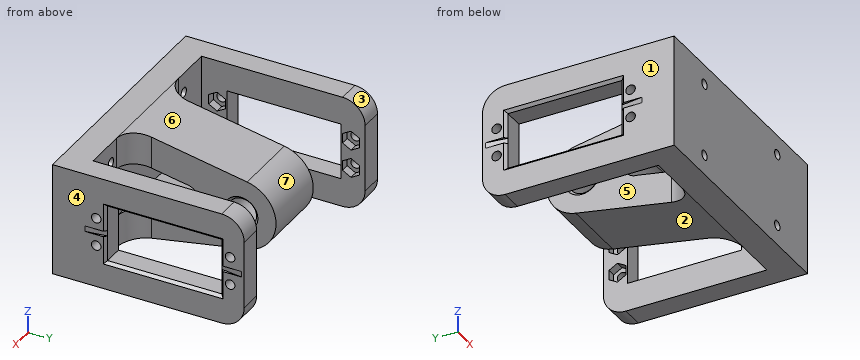
from build123d import *

# Parameters (mm, degrees)
SKETCH_1_W             = 8
SKETCH_1_H             = 58
SKETCH_1_W_2           = 12
EXTRUDE_1_DEPTH        = 20
SKETCH_3_R             = 1.7
SKETCH_3_W             = 20
SKETCH_3_H             = 40.5
CUT_EXTRUDE_1575_DEPTH = 8
SKETCH_2_R             = 5.05
CUT_EXTRUDE_2513_DEPTH = 12
CUT_EXTRUDE_2852_DEPTH = 1
SKETCH_5_R             = 1.7
CUT_EXTRUDE_3257_DEPTH = 3
SKETCH_6_R             = 1.7
CUT_EXTRUDE_5_DEPTH    = 10
FILLET_1_R             = 8
CHAMFER_1_SIZE         = 1


with BuildPart() as part:
    # Эскиз1 → Бобышка-Вытянуть1 (new body, symmetric)
    with BuildSketch(Plane.XY):
        Polygon((0, -10), (0, 0), (-12, 0), (-35, 0), (-43, 0), (-43, -10), align=None)
        with Locations((-39, 29)):
            Rectangle(SKETCH_1_W, SKETCH_1_H)
        with Locations((-6, 29)):
            Rectangle(SKETCH_1_W_2, SKETCH_1_H)
    extrude(amount=EXTRUDE_1_DEPTH, both=True)

    # Эскиз3 → Cut-Extrude 1575 (cut)
    with BuildSketch(Plane.ZY.offset(43)):
        with Locations((-5, 53)):
            Circle(SKETCH_3_R)
        with Locations((5, 53)):
            Circle(SKETCH_3_R)
        with Locations((-5, 5.5)):
            Circle(SKETCH_3_R)
        with Locations((5, 5.5)):
            Circle(SKETCH_3_R)
        with Locations((0, 29.25)):
            Rectangle(SKETCH_3_W, SKETCH_3_H)
    extrude(amount=-CUT_EXTRUDE_1575_DEPTH, mode=Mode.SUBTRACT)

    # Эскиз2 → Cut-Extrude 2513 (cut)
    with BuildSketch(Plane.ZY.offset(12)):
        with BuildLine():
            Line((-20, 58), (-20, 0))
            Line((-20, 0), (-12.294865589, 42.005278284))
            ThreePointArc((-12.294865589, 42.005278284), (0, 52.25), (12.294865589, 42.005278284))
            Line((12.294865589, 42.005278284), (20, 0))
            Line((20, 0), (20, 58))
            Line((20, 58), (-20, 58))
        make_face()
        with BuildLine():
            Line((-5, 20), (-8.668650572, 0))
            Line((-8.668650572, 0), (8.668650572, 0))
            Line((8.668650572, 0), (5, 20))
            ThreePointArc((5, 20), (0, 25), (-5, 20))
        make_face()
        with Locations((0, 39.75)):
            Circle(SKETCH_2_R)
    extrude(amount=-CUT_EXTRUDE_2513_DEPTH, mode=Mode.SUBTRACT)

    # Эскиз4 → Cut-Extrude 2852 (cut, symmetric)
    with BuildSketch(Plane.XY):
        Polygon((-42, 49.5), (-43, 49.5), (-43, 57), align=None)
        Polygon((-43, 9), (-43, 1.5), (-42, 9), align=None)
    extrude(amount=CUT_EXTRUDE_2852_DEPTH, both=True, mode=Mode.SUBTRACT)

    # Эскиз5 → Cut-Extrude 3257 (cut)
    with BuildSketch(Plane(origin=(-35, 0, 0), x_dir=(0, 0, -1), z_dir=(1, 0, 0))):
        Polygon((-6.732050808, 56), (-8.464101615, 53), (-6.732050808, 50), (-3.267949192, 50), (-1.535898385, 53), (-3.267949192, 56), align=None)
        with Locations((-5, 53)):
            Circle(SKETCH_5_R, mode=Mode.SUBTRACT)
        Polygon((1.535898385, 53), (3.267949192, 50), (6.732050808, 50), (8.464101615, 53), (6.732050808, 56), (3.267949192, 56), align=None)
        with Locations((5, 53)):
            Circle(SKETCH_5_R, mode=Mode.SUBTRACT)
        Polygon((-6.732050808, 8.5), (-8.464101615, 5.5), (-6.732050808, 2.5), (-3.267949192, 2.5), (-1.535898385, 5.5), (-3.267949192, 8.5), align=None)
        with Locations((-5, 5.5)):
            Circle(SKETCH_5_R, mode=Mode.SUBTRACT)
        Polygon((1.535898385, 5.5), (3.267949192, 2.5), (6.732050808, 2.5), (8.464101615, 5.5), (6.732050808, 8.5), (3.267949192, 8.5), align=None)
        with Locations((5, 5.5)):
            Circle(SKETCH_5_R, mode=Mode.SUBTRACT)
    extrude(amount=-CUT_EXTRUDE_3257_DEPTH, mode=Mode.SUBTRACT)

    # Эскиз6 → Вырез-Вытянуть5 (cut)
    with BuildSketch(Plane(origin=(0, 0, 0), x_dir=(1, 0, 0), z_dir=(0, 1, 0))):
        with Locations((-23.5, 13)):
            Circle(SKETCH_6_R)
        with Locations((-23.5, -13)):
            Circle(SKETCH_6_R)
    extrude(amount=-CUT_EXTRUDE_5_DEPTH, mode=Mode.SUBTRACT)

    # Скругление1
    fillet_1_edges = [part.edges().sort_by_distance(p)[0] for p in [
        (-39, 58, -20),
        (-12, 0, 14.334325286),
        (-39, 58, 20),
        (-12, 0, -14.334325286),
    ]]
    fillet(fillet_1_edges, radius=FILLET_1_R)

    # Фаска1
    chamfer_1_edges = [part.edges().sort_by_distance(p)[0] for p in [
        (-12, 39.75, -5.05),
        (-43, 9, 5.5),
        (-43, 49.5, 5.5),
        (-43, 29.25, 10),
        (-43, 9, -5.5),
        (-43, 49.5, -5.5),
        (-43, 29.25, -10),
    ]]
    chamfer(chamfer_1_edges, length=CHAMFER_1_SIZE)

    # Зеркальное отражение2: part across face


with BuildPart() as part_1:
    add(part.part)
    add(part.part.mirror(Plane(origin=(0, 17.029159437, 0), x_dir=(0, 0, 1), z_dir=(1, 0, 0))))


solid = part_1.part
The model under review builds one solid part; all positions refer to its coordinate system, in mm. Face numbers are marked on the shaded views. A direction names the side the tool comes from. Round coordinates to 2 decimals unless told otherwise and drop trailing zeros. Loops run counter-clockwise (first coordinate to the right, second up) from the corner with the lowest first, then second, coordinate; pieces in that order, holes last. Notation, with made-up numbers: (75, 62) -> (86, 62) arc R23 ccw to (86, 78) -> close; hole circle Ø3 at (70.25, 10.5). An arc over 180 degrees is marked (long way). Return JSON: item names as keys, results as strings.
(1) Add section D-D on z = 17. Write out the cut boundary in (x, y) (3 decimals), plus the area to 3 significant figures.
Solved:
{"outline": "(-43, -10) -> (43, -10) -> (43, 56.245) -> (35, 56.245) -> (35, 0) -> (20, 0) arc R8 cw to (12, 8) -> (12, 16.355) -> (-12, 16.355) -> (-12, 8) arc R8 cw to (-20, 0) -> (-35, 0) -> (-35, 56.245) -> (-43, 56.245) -> close", "area": "2,180 mm2"}
(2) For pin 1 (8 mm diameter, centred on y = 13.5, z = -4, fed in from -X); pin 2 (2.5 mm diameter, centred on x = -23.5, z = -13, fed in from +Y); pin 3 (1.5 mm diameter, centred on x = -22.5, z = -7.5, fed in from +Y), all flat-tipped, find the tip position at first contact; note any pin that passes through.
Solved:
{"pin 1": "x = -12", "pin 2": "through", "pin 3": "y = 0"}
(3) Add section A-A on z = 0. State how many separate pieces and enclosed holes the cut face has, plus the area to 3 significant figures.
Solved:
{"separate pieces": "5", "enclosed holes": "0", "area": "1,530 mm2"}
(4) For the marked faces 5, 6 and 7, list the 3-axis set-ups (+Z, -Z, +X, -X, +Y, -Y) from which the entire face can be reached by the end or side of a thin tool; tool diameter is ignored.
Solved:
{"face 5": "+Z, -Z, +Y", "face 6": "+Z, +Y", "face 7": "+Y"}
(5) The part is to be moulded in two halves that separate along X. For the marked faces 1, 2, 3 and 4, say which applies: released by +X, released by -X, zero draft, split by the parting line, or undercut.
Solved:
{"face 1": "released by -X", "face 2": "undercut", "face 3": "zero draft", "face 4": "released by +X"}
(6) Add section B-B on x = 23.5. Write out the cut boundary in (y, z).
Solved:
{"outline": "(-10, -20) -> (0, -20) -> (0, -14.7) -> (-10, -14.7) -> close; (-10, -11.3) -> (0, -11.3) -> (0, 11.3) -> (-10, 11.3) -> close; (-10, 14.7) -> (0, 14.7) -> (0, 20) -> (-10, 20) -> close"}
(7) Add section C-C on y = 11. Write out the cut boundary in (x, z).
Solved:
{"outline": "(-43, -20) -> (-35, -20) -> (-35, -10) -> (-42, -10) -> (-43, -11) -> close; (-43, 11) -> (-42, 10) -> (-35, 10) -> (-35, 20) -> (-43, 20) -> close; (-12, -17.98) -> (12, -17.98) -> (12, -6.65) -> (-12, -6.65) -> close; (-12, 6.65) -> (12, 6.65) -> (12, 17.98) -> (-12, 17.98) -> close; (35, -20) -> (43, -20) -> (43, -11) -> (42, -10) -> (35, -10) -> close; (35, 10) -> (42, 10) -> (43, 11) -> (43, 20) -> (35, 20) -> close"}
(8) For line 1 (Y direction, x = -39, z = -5); line 2 (Z direction, x = 23.5, y = -4.5); line 3 (X direction, y = 30, z = 11), list the stretches that pass through material, from the lowest coordinate up.
Solved:
{"line 1": "-10 to 3.8, 7.2 to 9, 49.5 to 51.3, 54.7 to 58", "line 2": "-20 to -14.7, -11.3 to 11.3, 14.7 to 20", "line 3": "-43 to -35, -12 to 12, 35 to 43"}
